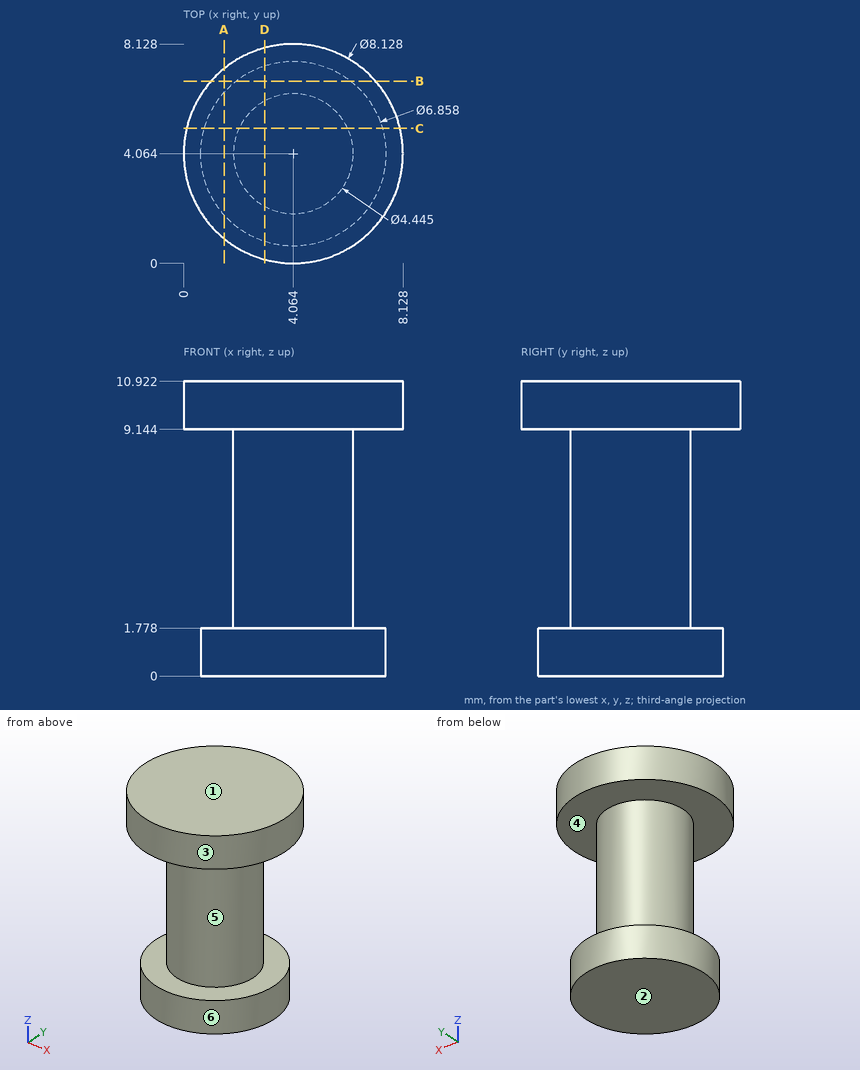
Here's the drawing with two shaded views (mm, measured from the low corner). I have some questions. A direction names the side the tool comes from. Round coordinates to 2 decimals unless told otherwise and drop trailing zeros. Write each loop counter-clockwise with the first axis right and the second up, starting at its lowest first coordinate (ties: lowest second). Pieces come first, ordered by that corner, then holes. Notation, with made-up numbers: M -27.5,5 L 3.5,5 A33 ccw 3.5,41 Z; hole C 15,47 d9. An arc over 180 degrees is marked long. Answer in a Markdown table with one row per item. Add a question column.
Q1. Imagine slicing it at C-C (y = 5). Please give me the cut outline in (x, z).
Q2. Imagine slicing it at A-A (x = 1.5). Please give me the cut outline in (y, z), then the cut area to 3 significant figures.
Q3. If we mould it in two halves opening along Z, with no side actions, what happens to the marked faces 1, 2, 3 and 4? For each: +Z half, -Z half, draft (parallel to the pull), parting line (faces both ways), or undercut.
Q4. Will these pins go through, and if not, where does the flat tip stop? pin 1 Ø4 at (y, z) = (2.5, 4) entering from -X; pin 2 Ø3 at (y, z) = (5, 1.5) entering from -X (3 decimals); pin 3 Ø4 at (y, z) = (1.5, 6) entering from +X.
Q5. On a 3-axis mill with a long thin cutter (end or side, diameter ignored), from which of +Z, -Z, +X, -X, +Y, -Y can I reach the whole of each face in a straight line? I mean the marked faces 5 and 6. Say none if no direction works.
Q6. Imagine slicing it at B-B (y = 6.75). Please give me the cut outline in (x, z), then the cut area to 3 significant figures.
Q7. Imagine slicing it at D-D (x = 3). Please give me the cut outline in (y, z), then the cut area to 3 significant figures.
Q8. If I drill on line 1 (Z direction, x = 0.75, y = 3.75); line 2 (X direction, y = 4, z = 2.5); line 3 (Z direction, x = 3.5, y = 7.5), over which ranges is the centre line in solid material (lowest first)? Write a range as from..to.
Values:
| question | item | result |
|---|---|---|
| 1 | outline | M 0.11,9.14 L 2.05,9.14 L 2.05,1.78 L 0.77,1.78 L 0.77,0 L 7.36,0 L 7.36,1.78 L 6.08,1.78 L 6.08,9.14 L 8.02,9.14 L 8.02,10.92 L 0.11,10.92 Z |
| 2 | outline | M 0.91,9.14 L 7.22,9.14 L 7.22,10.92 L 0.91,10.92 Z; M 1.79,0 L 6.34,0 L 6.34,1.78 L 1.79,1.78 Z |
| 2 | area | 19.3 mm^2 |
| 3 | face 1 | +Z half |
| 3 | face 2 | -Z half |
| 3 | face 3 | draft |
| 3 | face 4 | undercut |
| 4 | pin 1 | x = 1.84 |
| 4 | pin 2 | x = 0.635 |
| 4 | pin 3 | x = 6.21 |
| 5 | face 5 | none |
| 5 | face 6 | -Z |
| 6 | outline | M 1.01,9.14 L 7.11,9.14 L 7.11,10.92 L 1.01,10.92 Z; M 1.93,0 L 6.2,0 L 6.2,1.78 L 1.93,1.78 Z |
| 6 | area | 18.4 mm^2 |
| 7 | outline | M 0.14,9.14 L 2.11,9.14 L 2.11,1.78 L 0.8,1.78 L 0.8,0 L 7.32,0 L 7.32,1.78 L 6.02,1.78 L 6.02,9.14 L 7.99,9.14 L 7.99,10.92 L 0.14,10.92 Z |
| 7 | area | 54.3 mm^2 |
| 8 | line 1 | 0..1.78, 9.14..10.92 |
| 8 | line 2 | 1.84..6.29 |
| 8 | line 3 | 9.14..10.92 |
